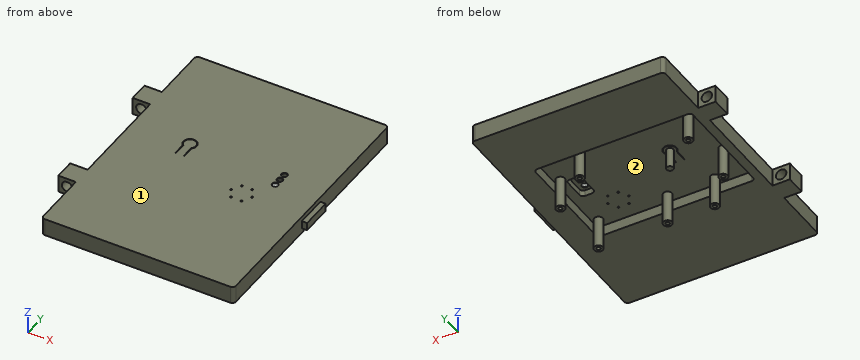
```python
from build123d import *

# Parameters (mm, degrees)
SKETCH1_W              = 110
SKETCH1_H              = 150
BOSS_EXTRUDE1_DEPTH    = 10
CUT_EXTRUDE1_DEPTH     = 6
SKETCH3_R              = 2.5
BOSS_EXTRUDE2_DEPTH    = 18
CUT_EXTRUDE2_START     = -12
SKETCH5_R              = 1.1
CUT_EXTRUDE2_DEPTH     = 5
CUT_EXTRUDE3_START     = 0.5
CUT_EXTRUDE3_DEPTH     = 4
SKETCH7_R              = 1.875
BOSS_EXTRUDE3_DEPTH    = 11.5
CUT_EXTRUDE4_DEPTH     = 4
SKETCH9_W              = 10
SKETCH9_H              = 11.4
BOSS_EXTRUDE4_DEPTH    = 10
SKETCH10_R             = 3
CUT_EXTRUDE5_DEPTH     = 161.819432905
SKETCH11_W             = 4.5
SKETCH11_H             = 18
BOSS_EXTRUDE5_DEPTH    = 3
FILLET1_R              = 2
CUT_EXTRUDE6_START     = -4
CUT_EXTRUDE6_OUTLINE_R = 0.5
CUT_EXTRUDE6_DEPTH     = 4


# Read off the part's stored shape, not the designer's step: Cut-Extrude6
with BuildPart() as part:
    # Sketch1 → Boss-Extrude1 (new body)
    with BuildSketch(Plane.XY):
        with Locations((55, 75)):
            Rectangle(SKETCH1_W, SKETCH1_H)
    extrude(amount=BOSS_EXTRUDE1_DEPTH)

    # Sketch2 → Cut-Extrude1 (cut)
    with BuildSketch(Plane(origin=(0, 0, 0), x_dir=(-1, 0, 0), z_dir=(0, 0, -1))):
        with BuildLine():
            Line((-93, 53), (-7, 53))
            ThreePointArc((-7, 53), (-5.585786438, 53.585786438), (-5, 55))
            Line((-5, 55), (-5, 113))
            ThreePointArc((-5, 113), (-5.585786438, 114.414213562), (-7, 115))
            Line((-7, 115), (-93, 115))
            ThreePointArc((-93, 115), (-94.414213562, 114.414213562), (-95, 113))
            Line((-95, 113), (-95, 55))
            ThreePointArc((-95, 55), (-94.414213562, 53.585786438), (-93, 53))
        make_face()
    extrude(amount=-CUT_EXTRUDE1_DEPTH, mode=Mode.SUBTRACT)

    # Sketch3 → Boss-Extrude2 (add)
    with BuildSketch(Plane(origin=(0, 0, 6), x_dir=(-1, 0, 0), z_dir=(0, 0, -1))):
        with Locations(Location((-91.46, 95.2, 0), (0, 0, 180))):
            Circle(SKETCH3_R)
        with Locations(Location((-70.96, 111.2, 0), (0, 0, 180))):
            Circle(SKETCH3_R)
        with Locations(Location((-9.46, 110.2, 0), (0, 0, 180))):
            Circle(SKETCH3_R)
        with Locations(Location((-9.46, 76.2, 0), (0, 0, 180))):
            Circle(SKETCH3_R)
        with Locations(Location((-24.96, 58.2, 0), (0, 0, 180))):
            Circle(SKETCH3_R)
        with Locations(Location((-51.96, 58.2, 0), (0, 0, 180))):
            Circle(SKETCH3_R)
        with Locations(Location((-91.46, 58.2, 0), (0, 0, 180))):
            Circle(SKETCH3_R)
    extrude(amount=BOSS_EXTRUDE2_DEPTH)

    # Sketch5 → Cut-Extrude2 (cut)
    with BuildSketch(Plane.XY.offset(CUT_EXTRUDE2_START)):
        with Locations(Location((91.46, 58.2, 0), (0, 0, 180))):
            Circle(SKETCH5_R)
        with Locations(Location((51.96, 58.2, 0), (0, 0, 180))):
            Circle(SKETCH5_R)
        with Locations(Location((24.96, 58.2, 0), (0, 0, 180))):
            Circle(SKETCH5_R)
        with Locations(Location((9.46, 76.2, 0), (0, 0, 180))):
            Circle(SKETCH5_R)
        with Locations(Location((9.46, 110.2, 0), (0, 0, 180))):
            Circle(SKETCH5_R)
        with Locations(Location((70.96, 111.2, 0), (0, 0, 180))):
            Circle(SKETCH5_R)
        with Locations(Location((91.46, 95.2, 0), (0, 0, 180))):
            Circle(SKETCH5_R)
    extrude(amount=CUT_EXTRUDE2_DEPTH, mode=Mode.SUBTRACT)

    # Sketch6 → Cut-Extrude3 (cut)
    with BuildSketch(Plane(origin=(0, 0, 6), x_dir=(-1, 0, 0), z_dir=(0, 0, -1)).offset(CUT_EXTRUDE3_START)):
        with BuildLine():
            Line((-87.5, 78), (-83.5, 78))
            ThreePointArc((-83.5, 78), (-82.085786438, 78.585786438), (-81.5, 80))
            Line((-81.5, 80), (-81.5, 91))
            ThreePointArc((-81.5, 91), (-82.085786438, 92.414213562), (-83.5, 93))
            Line((-83.5, 93), (-87.5, 93))
            ThreePointArc((-87.5, 93), (-88.914213562, 92.414213562), (-89.5, 91))
            Line((-89.5, 91), (-89.5, 80))
            ThreePointArc((-89.5, 80), (-88.914213562, 78.585786438), (-87.5, 78))
        make_face()
    extrude(amount=-CUT_EXTRUDE3_DEPTH, mode=Mode.SUBTRACT)

    # Sketch7 → Boss-Extrude3 (add)
    with BuildSketch(Plane(origin=(0, 0, 6), x_dir=(-1, 0, 0), z_dir=(0, 0, -1))):
        with Locations(Location((-32.95, 88.15, 0), (0, 0, 180))):
            Circle(SKETCH7_R)
    extrude(amount=BOSS_EXTRUDE3_DEPTH)

    # Sketch8 → Cut-Extrude4 (cut)
    with BuildSketch(Plane.XY.offset(10)):
        with BuildLine():
            Line((30.7, 78.15), (30.7, 85.469048676))
            ThreePointArc((30.7, 85.469048676), (32.95, 91.65), (35.2, 85.469048676))
            Line((35.2, 85.469048676), (35.2, 78.15))
            Line((35.2, 78.15), (35.5, 78.15))
            Line((35.5, 78.15), (35.5, 85.332643083))
            ThreePointArc((35.5, 85.332643083), (32.95, 91.95), (30.4, 85.332643083))
            Line((30.4, 85.332643083), (30.4, 78.15))
            Line((30.4, 78.15), (30.7, 78.15))
        make_face()
    extrude(amount=-CUT_EXTRUDE4_DEPTH, mode=Mode.SUBTRACT)

    # Sketch9 → Boss-Extrude4 (add)
    with BuildSketch(Plane.ZY):
        with Locations((5, 39)):
            Rectangle(SKETCH9_W, SKETCH9_H)
        with Locations((5, 111)):
            Rectangle(SKETCH9_W, SKETCH9_H)
    extrude(amount=BOSS_EXTRUDE4_DEPTH)

    # Sketch10 → Cut-Extrude5 (cut, through all)
    with BuildSketch(Plane(origin=(0, 116.7, 0), x_dir=(1, 0, 0), z_dir=(0, 1, 0))):
        with Locations(Location((-5, -5, 0), (0, 0, 270))):
            Circle(SKETCH10_R)
    extrude(amount=-CUT_EXTRUDE5_DEPTH, mode=Mode.SUBTRACT)

    # Sketch11 → Boss-Extrude5 (add)
    with BuildSketch(Plane(origin=(110, 0, 0), x_dir=(0, 0, -1), z_dir=(1, 0, 0))):
        with Locations((-5, 75)):
            Rectangle(SKETCH11_W, SKETCH11_H)
    extrude(amount=BOSS_EXTRUDE5_DEPTH)

    # Fillet1
    fillet1_edges = [part.edges().sort_by_distance(p)[0] for p in [
        (0, 150, 5),
        (110, 150, 5),
        (110, 0, 5),
        (0, 0, 5),
    ]]
    fillet(fillet1_edges, radius=FILLET1_R)

    # Cut-Extrude6 outline → Cut-Extrude6 (cut)
    with BuildSketch(Plane.XY.offset(10).offset(CUT_EXTRUDE6_START)):
        with BuildLine():
            add(Edge.make_bspline(
                [(83.934390614, 85.912779414), (83.934390614, 85.468732827), (84.302250852, 84.580639652), (85.634390614, 84.028849296), (86.966530376, 84.580639652), (87.518320733, 85.912779414), (86.966530376, 87.244919177), (85.634390614, 87.796709533), (84.302250852, 87.244919177), (83.934390614, 86.356826002), (83.934390614, 85.912779414)],
                knots=[0, 0, 0, 0, 0.125, 0.25, 0.375, 0.5, 0.625, 0.75, 0.875, 1, 1, 1, 1], degree=3))
        make_face()
        with BuildLine():
            add(Edge.make_bspline(
                [(83.948690614, 81.393579414), (83.948690614, 80.949532827), (84.316550852, 80.061439652), (85.648690614, 79.509649296), (86.980830376, 80.061439652), (87.532620733, 81.393579414), (86.980830376, 82.725719177), (85.648690614, 83.277509533), (84.316550852, 82.725719177), (83.948690614, 81.837626002), (83.948690614, 81.393579414)],
                knots=[0, 0, 0, 0, 0.125, 0.25, 0.375, 0.5, 0.625, 0.75, 0.875, 1, 1, 1, 1], degree=3))
        make_face()
        with BuildLine():
            add(Edge.make_bspline(
                [(83.934990614, 90.400579414), (83.934990614, 89.956532827), (84.302850852, 89.068439652), (85.634990614, 88.516649296), (86.967130376, 89.068439652), (87.518920733, 90.400579414), (86.967130376, 91.732719177), (85.634990614, 92.284509533), (84.302850852, 91.732719177), (83.934990614, 90.844626002), (83.934990614, 90.400579414)],
                knots=[0, 0, 0, 0, 0.125, 0.25, 0.375, 0.5, 0.625, 0.75, 0.875, 1, 1, 1, 1], degree=3))
        make_face()
        with Locations((68.959990614, 67.000579414)):
            Circle(CUT_EXTRUDE6_OUTLINE_R)
        with Locations((71.959990614, 72.196731837)):
            Circle(CUT_EXTRUDE6_OUTLINE_R)
        with Locations((77.959990614, 72.196731837)):
            Circle(CUT_EXTRUDE6_OUTLINE_R)
        with Locations((80.959990614, 67.000579414)):
            Circle(CUT_EXTRUDE6_OUTLINE_R)
        with Locations((77.959990614, 61.804426992)):
            Circle(CUT_EXTRUDE6_OUTLINE_R)
        with Locations((71.959990614, 61.804426992)):
            Circle(CUT_EXTRUDE6_OUTLINE_R)
    extrude(amount=CUT_EXTRUDE6_DEPTH, mode=Mode.SUBTRACT)


solid = part.part
```
Here's how the part is built. I have some questions about the finished solid (model axes, mm). Face numbers are marked on the shaded views. Coordinates: 2 decimals unless noted, no trailing zeros. Write each loop counter-clockwise with the first axis right and the second up, starting at its lowest first coordinate (ties: lowest second). Pieces come first, ordered by that corner, then holes. Notation, with made-up numbers: M 83,20 L 139,20 A20 cw 139,43 Z; hole C 41,21.25 d2. An arc over 180 degrees is marked long. Answer as CSV lines item,"result". Start each with the question number.
Q1. Suppose I cut it at A-A, the plane x = 46. List the corners of the cut face in (y, z) for me.
Q2. If we mould it in two halves opening along Y, with no side actions, what happens to the marked faces 1 and 2? For each: pulls with the +Y half, pulls with the -Y half, needs draft (parallel to the pull), parting line crosses it, or undercut.
Q3. Will these pins go through, and if not, where does the flat tip stop? pin 1 Ø1 at (y, z) = (86.5, 7.5) entering from -X; pin 2 Ø2.5 at (x, y) = (51.5, 58.5) entering from -Z; pin 3 Ø3 at (x, y) = (33.5, 89) entering from -Z; pin 4 Ø1 at (x, y) = (61, 78) entering from -Z.
Q4. Suppose I cut it at B-B, the plane y = 22. List the corners of the cut face in (x, z) for me.
Q5. I need wall thicknesses on probe 1 along Y at (x, z) = (91.46, -9.4); probe 2 along X at (y, z) = (58.2, -9.25); probe 3 along Y at (x, z) = (24.96, -8.65). Which ranges of each line are inside material? Lowest first, please. Write a range as [from, to].
Entries:
1,outline,"M 0,0 L 53,0 L 53,6 L 115,6 L 115,0 L 150,0 L 150,10 L 0,10 Z"
2,face 1,"needs draft"
2,face 2,"undercut"
3,pin 1,"stops at x = 0"
3,pin 2,"stops at z = -12"
3,pin 3,"stops at z = -5.5"
3,pin 4,"stops at z = 6"
4,outline,"M 0,0 L 110,0 L 110,10 L 0,10 Z"
5,probe 1,"y = [55.7, 57.1], [59.3, 60.7], [92.7, 94.1], [96.3, 97.7]"
5,probe 2,"x = [22.46, 23.86], [26.06, 27.46], [49.46, 50.86], [53.06, 54.46], [88.96, 90.36], [92.56, 93.96]"
5,probe 3,"y = [55.7, 57.1], [59.3, 60.7]"
